from build123d import *

# Parameters (mm, degrees)
SKETCH1_R           = 1.5
BOSS_EXTRUDE1_DEPTH = 5
SKETCH2_W           = 35
SKETCH2_H           = 2.5
BOSS_EXTRUDE2_DEPTH = 26
FILLET1_R           = 13
CUT_EXTRUDE1_DEPTH  = 13
SKETCH4_R           = 7.6
CUT_EXTRUDE2_DEPTH  = 1.2
SKETCH5_R           = 6.6
CUT_EXTRUDE3_DEPTH  = 50.27874954
CUT_EXTRUDE4_START  = 1.2
SKETCH6_R           = 7.6
CUT_EXTRUDE4_DEPTH  = 1.2
SKETCH7_R           = 6.6
CUT_EXTRUDE5_DEPTH  = 50.27874954
SKETCH8_R           = 4
CUT_EXTRUDE6_DEPTH  = 50.27874954


with BuildPart() as part:
    # Sketch1 → Boss-Extrude1 (new body)
    with BuildSketch(Plane(origin=(0, 0, 0), x_dir=(1, 0, 0), z_dir=(0, 1, 0))):
        Polygon((6, -10), (12.5, -10), (12.5, 0), (18.5, 0), (18.5, -10), (25, -10), (31, -10), (33, -10), (33, -36), (-2, -36), (-2, -10), (0, -10), align=None)
        with Locations(Location((15.5, -5, 0), (0, 0, 270))):
            Circle(SKETCH1_R, mode=Mode.SUBTRACT)
    extrude(amount=BOSS_EXTRUDE1_DEPTH)

    # Sketch2 → Boss-Extrude2 (add)
    with BuildSketch(Plane.XY.offset(36)):
        with Locations((15.5, 6.25)):
            Rectangle(SKETCH2_W, SKETCH2_H)
        with Locations((15.5, -1.25)):
            Rectangle(SKETCH2_W, SKETCH2_H)
    extrude(amount=-BOSS_EXTRUDE2_DEPTH)

    # Fillet1
    fillet1_edges = [part.edges().sort_by_distance(p)[0] for p in [
        (33, 2.5, 36),
        (-2, 2.5, 36),
    ]]
    fillet(fillet1_edges, radius=FILLET1_R)

    # Sketch3 → Cut-Extrude1 (cut)
    with BuildSketch(Plane(origin=(0, 0, 36), x_dir=(-1, 0, 0), z_dir=(0, 0, -1))):
        Polygon((-22.1, 7.5), (-22.1, 5.2875), (-23.1, 5.2875), (-23.1, 4.0875), (-15.5, 4.0875), (-7.9, 4.0875), (-7.9, 5.2875), (-8.9, 5.2875), (-8.9, 7.5), align=None)
    cut_extrude1 = extrude(amount=CUT_EXTRUDE1_DEPTH, mode=Mode.SUBTRACT)

    # Sketch4 → Cut-Extrude2 (cut)
    with BuildSketch(Plane(origin=(0, 4.0875, 0), x_dir=(1, 0, 0), z_dir=(0, 1, 0))):
        with Locations((15.5, -23)):
            Circle(SKETCH4_R)
    extrude(amount=CUT_EXTRUDE2_DEPTH, mode=Mode.SUBTRACT)

    # Sketch5 → Cut-Extrude3 (cut, through all)
    with BuildSketch(Plane(origin=(0, 4.0875, 0), x_dir=(1, 0, 0), z_dir=(0, 1, 0))):
        with Locations((15.5, -23)):
            Circle(SKETCH5_R)
    extrude(amount=CUT_EXTRUDE3_DEPTH, mode=Mode.SUBTRACT)

    # Mirror1: Cut-Extrude1 across plane
    add(cut_extrude1.mirror(Plane(origin=(0, 2.5, 0), x_dir=(0, 0, 1), z_dir=(0, -1, 0))), mode=Mode.SUBTRACT)

    # Sketch6 → Cut-Extrude4 (cut)
    with BuildSketch(Plane.XZ.offset(-0.9125).offset(CUT_EXTRUDE4_START)):
        with Locations((15.5, 23)):
            Circle(SKETCH6_R)
    extrude(amount=-CUT_EXTRUDE4_DEPTH, mode=Mode.SUBTRACT)

    # Sketch7 → Cut-Extrude5 (cut, through all)
    with BuildSketch(Plane.XZ.offset(-0.9125)):
        with Locations((15.5, 23)):
            Circle(SKETCH7_R)
    extrude(amount=CUT_EXTRUDE5_DEPTH, mode=Mode.SUBTRACT)

    # Sketch8 → Cut-Extrude6 (cut, through all)
    with BuildSketch(Plane(origin=(0, 4.0875, 0), x_dir=(1, 0, 0), z_dir=(0, 1, 0))):
        with Locations(Location((15.5, -23, 0), (0, 0, 270))):
            Circle(SKETCH8_R)
    extrude(amount=-CUT_EXTRUDE6_DEPTH, mode=Mode.SUBTRACT)


solid = part.part
Verification items for the finished model (mm, model axes). A direction names the side the tool comes from. Give positions to 0.01 mm unless a question says otherwise; leave off trailing zeros. Write each loop counter-clockwise with the first axis right and the second up, starting at its lowest first coordinate (ties: lowest second). Pieces come first, ordered by that corner, then holes. Notation, with made-up numbers: M 11.25,-29 L 20.25,-29 A16 cw 20.25,-18 Z; hole C 5,39 d1. An arc over 180 degrees is marked long. Put each result on its own line as item: value. Start each with the question number.
1. Draft check along Z on faces 1 (the face through (18.2, 2.52, 20.05)), 2 (the face through (22.1, -1, 30)), 3 (the face through (15, 3, 36)). Enter one of: +Z half, -Z half, draft (parallel to the pull), parting line (faces both ways), or undercut.
2. Set-up check for faces 4 (the face through (18.5, 2, 5)), 5 (the face through (16, 0.912, 28)), 6 (the face through (22.1, 6, 30)), 7 (the face through (12.5, 2, 5)): record each of +Z, -Z, +X, -X, +Y, -Y from which the full face is reachable in a straight line by a thin tool's end or side.
3. Section check C-C (y = 3.25). Record the cut outline in (x, z), and give its area (3 significant figures).
4. Section check A-A (x = 15.5). Record the cut outline in (y, z).
5. Section check D-D (z = 18). Record the cut outline in (x, y), and give its area (3 significant figures).
6. Section check B-B (z = 5). Record the cut outline in (x, y), and give its area (3 significant figures).
7. Scan lines: line 1 along X through (y, z) = (2.8, 23); line 2 along X through (y, z) = (-1.25, 23); line 3 along Y through (x, z) = (14, 27.5). Record each from-to range of solid material in increasing order. Write a range as [from, to].
8. Go/stop test with flat-tipped pins: pin 1 Ø1.1 at (y, z) = (6.5, 31.5) entering from -X; pin 2 Ø6.5 at (x, z) = (17, 3) entering from +Y; pin 3 Ø1 at (y, z) = (5, 31.5) entering from -X; pin 4 Ø5 at (x, y) = (11.5, 4) entering from -Z. Record where each tip stops, or that it passes through.
Answer list:
1. face 1: undercut
1. face 2: draft
1. face 3: +Z half
2. face 4: -Z, +X, +Y, -Y
2. face 5: +Z
2. face 6: +Z, +Y
2. face 7: -Z, -X, +Y, -Y
3. outline: M -2,10 L 12.5,10 L 12.5,0 L 18.5,0 L 18.5,10 L 33,10 L 33,23 A13 ccw 20,36 L 11,36 A13 ccw -2,23 Z; hole C 15.5,23 d8; hole C 15.5,5 d3
3. area: 840 mm2
4. outline: M -2.5,10 L 0,10 L 0,6.5 L 5,6.5 L 5,10 L 7.5,10 L 7.5,16.4 L 5.29,16.4 L 5.29,15.4 L 4.09,15.4 L 4.09,19 L 0.91,19 L 0.91,15.4 L -0.29,15.4 L -0.29,16.4 L -2.5,16.4 Z; M 0,0 L 5,0 L 5,3.5 L 0,3.5 Z; M 0.91,27 L 4.09,27 L 4.09,36 L 0.91,36 Z
5. outline: M -2,-2.5 L 11.19,-2.5 L 11.19,-0.29 L 9.78,-0.29 L 9.78,0.91 L 21.22,0.91 L 21.22,-0.29 L 19.81,-0.29 L 19.81,-2.5 L 33,-2.5 L 33,7.5 L 19.81,7.5 L 19.81,5.29 L 21.22,5.29 L 21.22,4.09 L 9.78,4.09 L 9.78,5.29 L 11.19,5.29 L 11.19,7.5 L -2,7.5 Z
5. area: 284 mm2
6. outline: M 12.5,0 L 14,0 L 14,5 L 12.5,5 Z; M 17,0 L 18.5,0 L 18.5,5 L 17,5 Z
6. area: 15.0 mm2
7. line 1: [-2, 11.5], [19.5, 33]
7. line 2: [-2, 8.9], [22.1, 33]
7. line 3: [0.91, 4.09]
8. pin 1: x = 0.71
8. pin 2: y = 5
8. pin 3: x = 0.75
8. pin 4: z = 0
